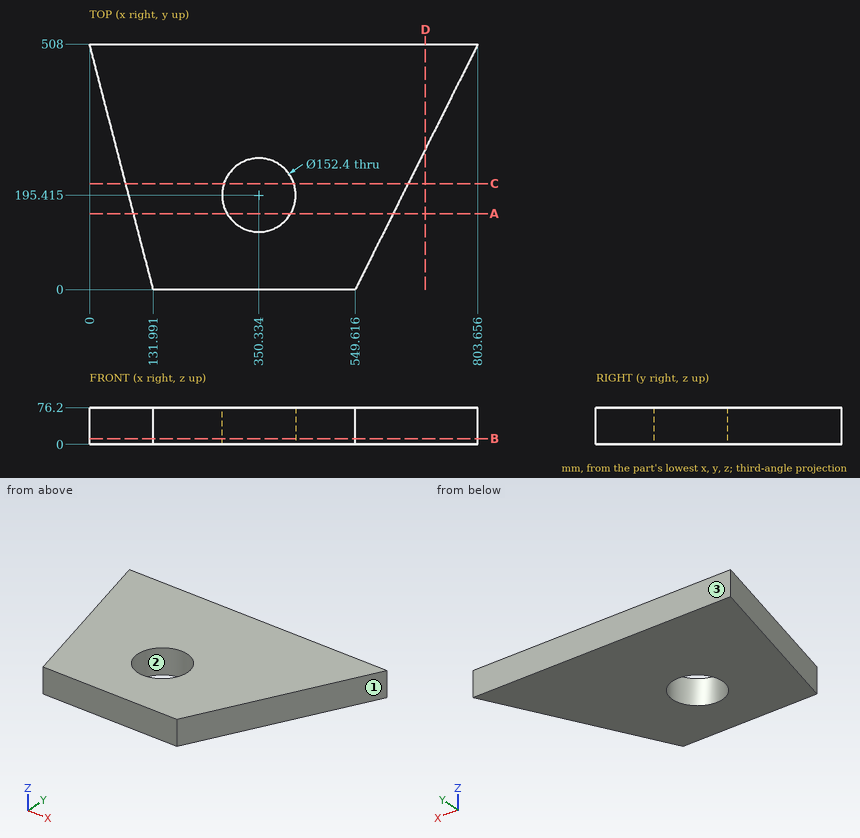
The figure shows three views and two pictorial views of one solid part (mm, origin at its lowest corner). Answer the questions. Round coordinates to 2 decimals unless told otherwise and drop trailing zeros. Order: outer loops, then holes, each group sorted by start corner. A loop starts at its lowest first (then second) coordinate and runs counter-clockwise, first axis right, second up.
Q1. A cutting plane is placed at A-A, the plane y = 157. Determine the outline of the cut face in (x, z).
Solution:
outline: (91.2, 0) - (284.53, 0) - (284.53, 76.2) - (91.2, 76.2) - close; (416.14, 0) - (628.13, 0) - (628.13, 76.2) - (416.14, 76.2) - close
Q2. Given pin 1 Ø1 at (y, z) = (296.5, 39.5) entering from -X; pin 2 Ø4 at (y, z) = (204, 54) entering from -X; pin 3 Ø10 at (y, z) = (200.5, 32) entering from -X, each flat-ended and moving along its own axis, determine where each tip first touches the part or whether it passes through.
Solution:
pin 1: stops at x = 54.82
pin 2: stops at x = 78.47
pin 3: stops at x = 78.6
Q3. Find the intervals of material crossed by line 1 along X through (y, z) = (175, 65); line 2 along Y through (x, z) = (314.5, 68); line 3 along X through (y, z) = (364.5, 69) (1 decimal), in increasing order.
Solution:
line 1: x = 86.52 to 276.92, 423.75 to 637.13
line 2: y = 0 to 128.17, 262.66 to 508
line 3: x = 37.3 to 731.9
Q4. A cutting plane is placed at D-D, the plane x = 695. Determine the outline of the cut face in (y, z).
Solution:
outline: (290.72, 0) - (508, 0) - (508, 76.2) - (290.72, 76.2) - close
Q5. A cutting plane is placed at C-C, the plane y = 219. Determine the outline of the cut face in (x, z), then the cut area to 3 significant figures.
Solution:
outline: (75.09, 0) - (277.88, 0) - (277.88, 76.2) - (75.09, 76.2) - close; (422.79, 0) - (659.13, 0) - (659.13, 76.2) - (422.79, 76.2) - close
area: 33,500 mm2
Q6. A cutting plane is placed at B-B, the plane z = 12. Determine the outline of the cut face in (x, y) (1 decimal).
Solution:
outline: (0, 508) - (132, 0) - (549.6, 0) - (803.7, 508) - close; hole circle Ø152.4 at (350.3, 195.4)
Q7. The mould has two halves that part along Y. Classify the marked faces 1, 2 and 3: pulls with the +Y half, pulls with the -Y half, needs draft (parallel to the pull), parting line crosses it, or undercut.
Solution:
face 1: pulls with the -Y half
face 2: undercut
face 3: pulls with the +Y half
